```python
from build123d import *

# Parameters (mm, degrees)
F1_DEPTH      = 25
F1_DEPTH_BACK = 25


with BuildPart() as f1:
    # F0 (on Front) → F1 (new body, two sides)
    with BuildSketch(Plane.XZ) as f1_sk:
        Polygon((-42.7725724876, 38.9332138002), (0, 0), (34.5220863819, 0), (34.5220863819, 25.2119097859), (-18.3541122824, 25.2119097859), (-18.3541122824, 46.9000972807), (33.7701886892, 46.9000972807), (33.7701886892, 71.300983429), (0, 71.300983429), align=None)
    extrude(amount=-F1_DEPTH)
    extrude(f1_sk.sketch, amount=F1_DEPTH_BACK)


solid = f1.part
```
Can you work these out from the model? Positions are in its coordinate system, mm. A direction names the side the tool comes from. Round coordinates to 2 decimals unless told otherwise and drop trailing zeros. Loops run counter-clockwise (first coordinate to the right, second up) from the corner with the lowest first, then second, coordinate; pieces in that order, holes last. Notation, with made-up numbers: M 66.5,53 L 71.5,53 A20 cw 71.5,75 Z; hole C 72.5,75.25 d2. An arc over 180 degrees is marked long. Answer as a JSON object with one key per item and string values. Group by question number.
Q1. Please list where these lines run through material, in increasing order: L1, parallel to Z at x = 6.5, y = -0.5; L2, parallel to Z at x = -20, y = -2; L3, parallel to X at y = 8, z = 38.5.
Q2. We'd pull the mould along Z, two halves only. Please class faces 4 (the flat face through (4, 25, 20)), 5 (the flat face through (-21.686, 0.35, 19.739)), 6 (the flat face through (17, 0, 71.301)), 7 (the flat face through (8, 0, 25.212)): +Z half, -Z half, draft (parallel to the pull), parting line (faces both ways), or undercut.
Q3. Imagine slicing it at D-D, the plane z = 22. Please give me the cut outline in (x, y), then the cut area to 3 significant figures.
Q4. Imagine slicing it at C-C, the plane x = -17. Please give me the cut outline in (y, z), then the cut area to 3 significant figures.
Q5. Imagine slicing it at A-A, the plane x = 12. Please give me the cut outline in (y, z), then the cut area to 3 significant figures.
Q6. On a 3-axis mill with a long thin cutter (end or side, diameter ignored), from which of +Z, -Z, +X, -X, +Y, -Y can I reach the whole of each face in a straight line? I mean faces 1 (the flat face through (33.77, 0, 59)), 2 (the flat face through (17, 0, 0)), 3 (the flat face through (-18.354, 0, 36)). Say none if no direction works.
Q7. Will these pins go through, and if not, where does the flat tip stop? pin 1 (8 mm diameter, centred on y = -0.5, z = 35.5, fed in from -X); pin 2 (6 mm diameter, centred on y = -3, z = 57, fed in from -X); pin 3 (3 mm diameter, centred on y = 6.5, z = 14, fed in from -X).
Q8. Imagine slicing it at B-B, the plane y = 20.5. Please give me the cut outline in (x, z), then the cut area to 3 significant figures.
Findings:
{
 "1": {"L1": "z = 0 to 25.21, 46.9 to 71.3", "L2": "z = 18.2 to 56.17", "L3": "x = -42.3 to -18.35"},
 "2": {"face 4": "draft", "face 5": "-Z half", "face 6": "+Z half", "face 7": "undercut"},
 "3": {"outline": "M -24.17,-25 L 34.52,-25 L 34.52,25 L -24.17,25 Z", "area": "2,930 mm2"},
 "4": {"outline": "M -25,15.47 L 25,15.47 L 25,25.21 L -25,25.21 Z; M -25,46.9 L 25,46.9 L 25,58.44 L -25,58.44 Z", "area": "1,060 mm2"},
 "5": {"outline": "M -25,0 L 25,0 L 25,25.21 L -25,25.21 Z; M -25,46.9 L 25,46.9 L 25,71.3 L -25,71.3 Z", "area": "2,480 mm2"},
 "6": {"face 1": "+Z, +X, +Y, -Y", "face 2": "-Z, +X, -X, +Y, -Y", "face 3": "+X, +Y, -Y"},
 "7": {"pin 1": "stops at x = -42.77", "pin 2": "stops at x = -22.86", "pin 3": "stops at x = -17.03"},
 "8": {"outline": "M -42.77,38.93 L 0,0 L 34.52,0 L 34.52,25.21 L -18.35,25.21 L -18.35,46.9 L 33.77,46.9 L 33.77,71.3 L 0,71.3 Z", "area": "2,820 mm2"}
}
